Work out the finished part from the listing and answer in its coordinate system (mm). Face numbers are marked on the shaded views. A direction names the side the tool comes from. Round coordinates to 2 decimals unless told otherwise and drop trailing zeros. Order: outer loops, then holes, each group sorted by start corner. A loop starts at its lowest first (then second) coordinate and runs counter-clockwise, first axis right, second up. Notation, with made-up numbers: (-11.75, 67) - (31.25, 67) arc R26 cw to (31.25, 103) - close; hole circle Ø5 at (-26, -37.75). An arc over 180 degrees is marked (long way). Use CSV: the item, a comma, the result in double quotes.
from build123d import *

# Parameters (mm, degrees)
F1_DEPTH = 20
F2_START = 1.5
F2_DEPTH = 17
F3_W     = 17
F3_H     = 17
F4_DEPTH = 30
F5_W     = 17
F5_H     = 17
F6_DEPTH = 30
F7_W     = 17
F7_H     = 17
F8_DEPTH = 30


with BuildPart() as f1:
    # F0 (on Top) → F1 (new body)
    with BuildSketch(Plane.XY):
        Polygon((8.5, -10), (10, -10), (10, 10), (-10, 10), (-10, 8.5), (-10, 0), (-10, -8.5), (-10, -10), (-8.5, -10), (0, -10), align=None)
    extrude(amount=F1_DEPTH)

    # F0 (on Top) → F2 (join)
    with BuildSketch(Plane.XY.offset(F2_START)):
        Polygon((-10, 0), (-10, 8.5), (-40, 8.5), (-40, -8.5), (-10, -8.5), align=None)
        Polygon((8.5, -40), (8.5, -10), (0, -10), (-8.5, -10), (-8.5, -40), align=None)
    extrude(amount=F2_DEPTH)

    # F3 (on face) → F4 (join)
    with BuildSketch(Plane.XY.offset(20)):
        Rectangle(F3_W, F3_H)
    extrude(amount=F4_DEPTH)

    # F5 (on face) → F6 (join)
    with BuildSketch(Plane(origin=(0, 0, 0), x_dir=(1, 0, 0), z_dir=(0, 0, -1))):
        Rectangle(F5_W, F5_H)
    extrude(amount=F6_DEPTH)

    # F7 (on face) → F8 (join)
    with BuildSketch(Plane.YZ.offset(10)):
        with Locations((0, 10)):
            Rectangle(F7_W, F7_H)
    extrude(amount=F8_DEPTH)


solid = f1.part
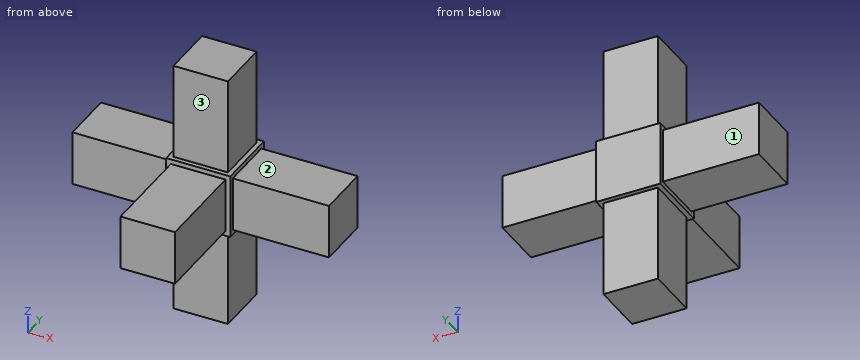
(1) Find section C-C (z = 14.5). Determine the outline of the cut face in (x, y), and give its area (3 significant figures).
Findings below:
outline,"(-40, -8.5) - (-10, -8.5) - (-10, -10) - (-8.5, -10) - (-8.5, -40) - (8.5, -40) - (8.5, -10) - (10, -10) - (10, -8.5) - (40, -8.5) - (40, 8.5) - (10, 8.5) - (10, 10) - (-10, 10) - (-10, 8.5) - (-40, 8.5) - close"
area,"1,930 mm²"
(2) Find section B-B (y = 0). Determine the outline of the cut face in (x, z).
Findings below:
outline,"(-40, 1.5) - (-10, 1.5) - (-10, 0) - (-8.5, 0) - (-8.5, -30) - (8.5, -30) - (8.5, 0) - (10, 0) - (10, 1.5) - (40, 1.5) - (40, 18.5) - (10, 18.5) - (10, 20) - (8.5, 20) - (8.5, 50) - (-8.5, 50) - (-8.5, 20) - (-10, 20) - (-10, 18.5) - (-40, 18.5) - close"
(3) Find the intervals of material crossed by L1, parallel to Z at x = 5, y = -24; L2, parallel to Y at x = 2, z = 30, in increasing order. Write a range as from..to.
Findings below:
L1,"z = 1.5..18.5"
L2,"y = -8.5..8.5"
(4) Find section A-A (x = -2). Determine the outline of the cut face in (y, z), and give its area (3 significant figures).
Findings below:
outline,"(-40, 1.5) - (-10, 1.5) - (-10, 0) - (-8.5, 0) - (-8.5, -30) - (8.5, -30) - (8.5, 0) - (10, 0) - (10, 20) - (8.5, 20) - (8.5, 50) - (-8.5, 50) - (-8.5, 20) - (-10, 20) - (-10, 18.5) - (-40, 18.5) - close"
area,"1,930 mm²"
(5) Find section D-D (z = -4). Determine the outline of the cut face in (x, y).
Findings below:
outline,"(-8.5, -8.5) - (8.5, -8.5) - (8.5, 8.5) - (-8.5, 8.5) - close"
(6) For the marked faces 1, 2 and 3, determine the directions among +Z, -Z, +X, -X, +Y, -Y from which every point of the face is accessible in a straight line to the end or side of a thin tool.
Findings below:
face 1,"+Z, -Z, -X, +Y"
face 2,"+Z, +X, +Y, -Y"
face 3,"+Z, +X, -X, -Y"
(7) Each of these flat-tipped pins is pushed along its axis until it touches: pin 1 (1.5 mm diameter, centred on x = -3, y = -11, fed in from +Z); pin 2 (18.5 mm diameter, centred on x = 0, z = -8.5, fed in from -Y); pin 3 (13.5 mm diameter, centred on x = 0, z = 38, fed in from -Y). Where does it stop, or does it pass through?
Findings below:
pin 1,"stops at z = 18.5"
pin 2,"stops at y = -10"
pin 3,"stops at y = -8.5"
